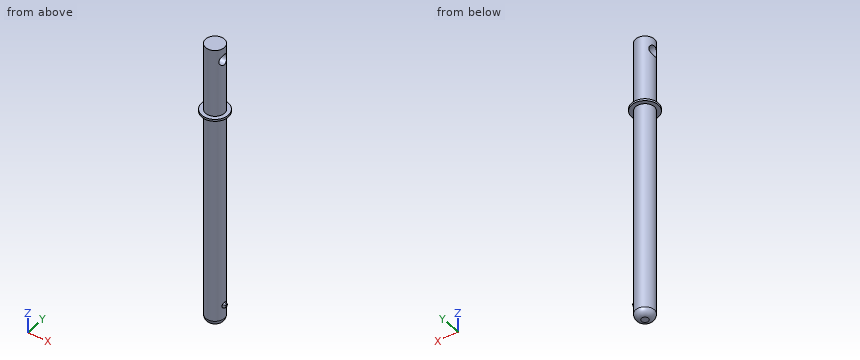
Autodesk Inventor part; units mm, degrees
ref_plane "Work Plane1" through (5, 0, 0) normal (1, 0, 0) x (0, 1, 0)
ref_plane "XZ Plane" through (0, 0, 0) normal (0, 1, 0) x (-1, 0, 0)
ref_plane "XY Plane" through (0, 0, 0) normal (0, 0, 1) x (1, 0, 0)
sketch "Sketch1" plane through (0, 0, 0) normal (0, 0, 1) x (1, 0, 0)
  circle A0 centre (0, 0) radius 2.38125
  dimension "d0" = 4.7625
extrude "Extrusion1" add sketch "Sketch1" along normal blind 73.3298
ref_plane "Work Plane1" through (5, 0, 0) normal (1, 0, 0) x (0, 1, 0)
sketch "Sketch2" plane through (5, 0, 0) normal (1, 0, 0) x (0, 1, 0)
  line L0 (-2.38125, 73.3298) -> (2.38125, 73.3298)
  line L1 (-2.38125, 0) -> (2.38125, 0)
  line L2 (-2.38125, 0) -> (-2.38125, 73.3298)
  line L3 (2.38125, 0) -> (2.38125, 73.3298)
  circle A0 centre (0, 70.142643) radius 1.35
  point P0 (0, 0)
  dimension "d4" = 2.7
extrude "Extrusion2" cut sketch "Sketch2" against normal blind 39.4202 contours A0
sketch "Sketch3" plane through (0, 0, 0) normal (1, 0, 0) x (0, 1, 0)
  arc A0 (-1.35, 70.142643) -> (-1.35, 70.142643) centre (-1.35, 70.142643) ccw
  arc A1 (-1.35, 70.142643) -> (-1.35, 70.142643) centre (-1.35, 70.142643) ccw
  line L0 (-2.38125, 73.3298) -> (2.38125, 73.3298)
  line L1 (-2.38125, 0) -> (2.38125, 0)
  line L2 (2.38125, 0) -> (2.38125, 73.3298)
  line L3 (-2.38125, 0) -> (-2.38125, 73.3298)
  line L4 (2.38125, 55.88) -> (3.38125, 55.88)
  line L5 (3.38125, 55.88) -> (3.38125, 55.38)
  line L6 (3.38125, 55.38) -> (2.38125, 55.38)
  line L7 (2.38125, 55.38) -> (2.38125, 55.88)
  line L8 (0, -14.66596) -> (0, 87.99576)
  point P0 (0, 0)
  dimension "d7" = 1
  dimension "d8" = 0.5
  dimension "d9" = 17.4498
sketch "Sketch3 outline for Revolution1" plane through (0, 0, 0) normal (1, 0, 0) x (0, 1, 0)
  line L0 (3.38125, 55.88) -> (2.38125, 55.88)
  line L1 (3.38125, 55.38) -> (3.38125, 55.88)
  line L2 (2.38125, 55.38) -> (3.38125, 55.38)
  line L3 (2.38125, 55.88) -> (2.38125, 55.38)
revolve "Revolution1" add sketch "Sketch3 outline for Revolution1" angle 360 about axis through (0, 0, -10) along (0, 0, 1)
sketch "Sketch4" plane through (0, 0, 0) normal (1, 0, 0) x (0, 1, 0)
  circle A0 centre (0, 5.08) radius 0.7
  point P0 (0, 0)
  dimension "d11" = 1.4
  dimension "d12" = 5.08
extrude "Extrusion3" add sketch "Sketch4" along normal blind 2.9202
fillet "Fillet1" radius 0.6 1 edges at (2.9202, -0.7, 5.08)
fillet "Fillet2" radius 1.5 1 edges at (-2.3813, 0, 0)
properties part number "launcher.RBFpin"
Work out the finished part from the listing and answer in its coordinate system (mm). Round coordinates to 2 decimals unless told otherwise and drop trailing zeros. Write each loop counter-clockwise with the first axis right and the second up, starting at its lowest first coordinate (ties: lowest second). Pieces come first, ordered by that corner, then holes.
1) Straight lines are drawn through the part: line 1 (Z direction, x = -0.2, y = 0); line 2 (Z direction, x = -2.5, y = 1.75); line 3 (X direction, y = -0.25, z = 51). For each, find the intervals that lie inside material, in ascending order.
2) Given pin 1 Ø2 at (x, z) = (-2, 47.5) entering from -Y; pin 2 Ø1.5 at (x, y) = (-2, -2.5) entering from -Z; pin 3 Ø3 at (x, z) = (0.5, 17) entering from -Y, each flat-ended and moving along its own axis, determine where each tip first touches the part or whether it passes through.
3) A cutting plane is placed at A-A (z = 28.5). Give the vertices of the cut face in (x, y), plus the area to 3 significant figures.
Completed:
1. line 1: z = 0 to 68.79, 71.49 to 73.33
1. line 2: z = 55.38 to 55.88
1. line 3: x = -2.37 to 2.37
2. pin 1: stops at y = -2.16
2. pin 2: stops at z = 55.38
2. pin 3: stops at y = -2.38
3. outline: circle Ø4.76 at (0, 0)
3. area: 17.8 mm2
